Read the model definition and answer for the solid it produces. Units are mm, in the model's axes. A direction names the side the tool comes from. Give positions to 0.01 mm unless a question says otherwise; leave off trailing zeros. Loops run counter-clockwise (first coordinate to the right, second up) from the corner with the lowest first, then second, coordinate; pieces in that order, holes last. Notation, with made-up numbers: (-32.5, 78.5) -> (-20.5, 78.5) arc R18 ccw to (-20.5, 89.5) -> close; hole circle Ø7 at (34, 56). An arc over 180 degrees is marked (long way). Write each question's results on one line, items separated by ' | '. Start each with the question number.
Item 1: Section C-C on y = 24 is taken. Write down the section's boundary in (x, z).
Item 2: Find the intervals of material crossed by line 1 (Z direction, x = 7.5, y = 25.25); line 2 (Z direction, x = 5, y = 7.75); line 3 (Y direction, x = 5, z = 6.75), in increasing order.
Item 3: Which of the six approach directions +Z, -Z, +X, -X, +Y, -Y give full straight-line access (tool end or side, diameter ignored) to faces 4 (the flat face through (15, 16, 2)), 5 (the flat face through (5.7, 23, 7.4))?
Item 4: Each of these flat-tipped pins is pushed along its axis until it touches: P1, Ø7.5, axis at x = 4.5, y = 7, coming from the +Z side; P2, Ø6, axis at x = 6.5, z = 8, coming from the -Y side. Where does it stop, or does it pass through?
Item 5: Section D-D on x = 3.5 is taken. Write down the section's boundary in (y, z), and give its area (3 significant figures).
Item 6: Section B-B on z = 7.5 is taken. Write down the section's boundary in (x, y), and give its area (3 significant figures).
Item 7: Determine the mould class of faces 1 (the flat face through (7, 25, 12)), 2 (the cylindrical face through (7.85, 24.52, 5.94)), 3 (the flat face through (7, 26, 5)) for opening direction Z: +Z half, -Z half, draft (parallel to the pull), parting line (faces both ways), or undercut.
Item 8: Section A-A on x = 7.5 is taken. Write down the section's boundary in (y, z).
```python
from build123d import *

# Parameters (mm, degrees)
F0_W     = 15
F0_H     = 23
F1_DEPTH = 3
F0_H_2   = 3
F2_DEPTH = 12
F4_D     = 3.2


with BuildPart() as f1:
    # F0 (on Top) → F1 (new body)
    with BuildSketch(Plane.XY):
        with Locations((7.5, 11.5)):
            Rectangle(F0_W, F0_H)
    extrude(amount=F1_DEPTH)

    # F0 (on Top) → F2 (join)
    with BuildSketch(Plane.XY):
        with Locations((7.5, 24.5)):
            Rectangle(F0_W, F0_H_2)
    extrude(amount=F2_DEPTH)

    # F4 (through all)
    with Locations(Plane.XZ.offset(-23)):
        with Locations((7.5, 7.5)):
            Hole(F4_D / 2)


solid = f1.part
```
Findings:
1) outline: (0, 0) -> (15, 0) -> (15, 12) -> (0, 12) -> close; hole circle Ø3.2 at (7.5, 7.5)
2) line 1: 0 to 5.9, 9.1 to 12 | line 2: 0 to 3 | line 3: 23 to 26
3) face 4: +Z, -Z, +X, +Y, -Y | face 5: +Z, +X, -X, -Y
4) P1: z = 3 | P2: y = 23
5) outline: (0, 0) -> (26, 0) -> (26, 12) -> (23, 12) -> (23, 3) -> (0, 3) -> close | area: 105 mm2
6) outline: (0, 23) -> (5.9, 23) -> (5.9, 26) -> (0, 26) -> close; (9.1, 23) -> (15, 23) -> (15, 26) -> (9.1, 26) -> close | area: 35.4 mm2
7) face 1: +Z half | face 2: undercut | face 3: draft
8) outline: (0, 0) -> (26, 0) -> (26, 5.9) -> (23, 5.9) -> (23, 3) -> (0, 3) -> close; (23, 9.1) -> (26, 9.1) -> (26, 12) -> (23, 12) -> close
